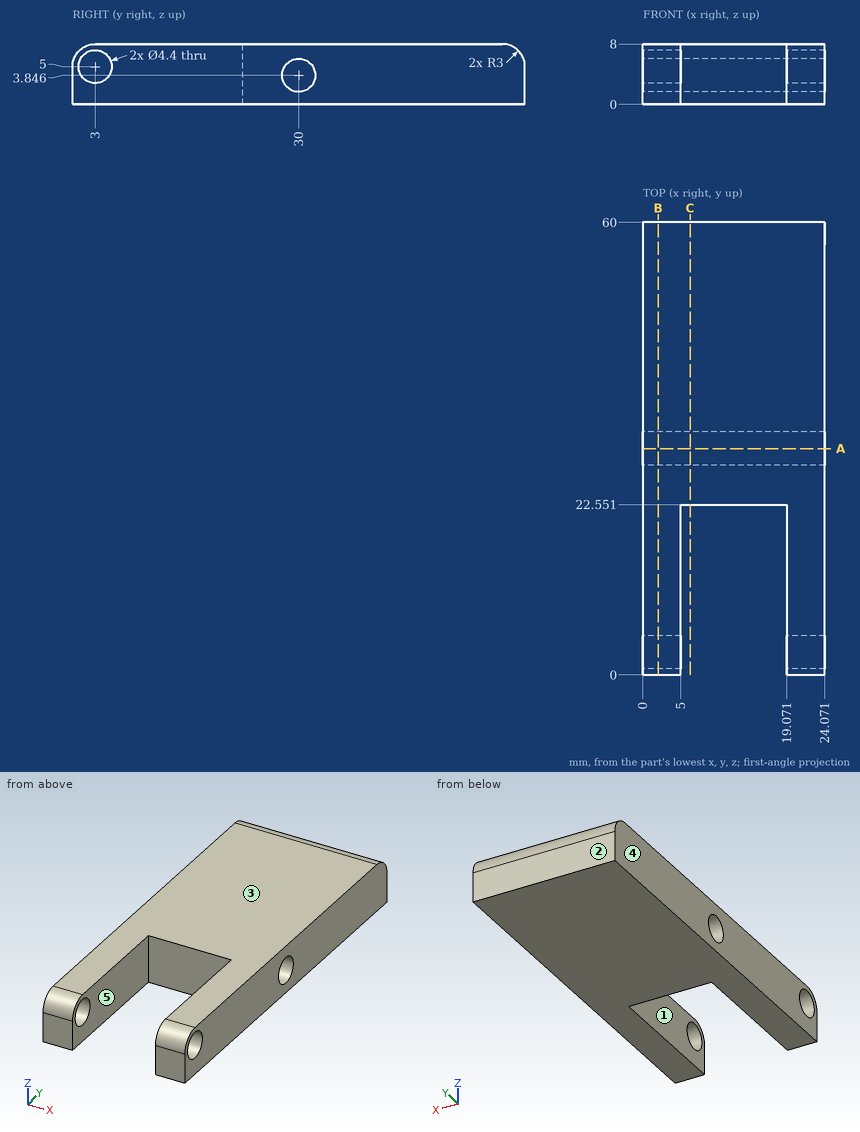
Answer from the drawing. Dimensions are ordinates in mm from the lowest x, y and z of the part. A direction names the side the tool comes from. Round coordinates to 2 decimals unless told otherwise and drop trailing zeros. Order: outer loops, then holes, each group sorted by start corner. A loop starts at its lowest first (then second) coordinate and runs counter-clockwise, first axis right, second up. Notation, with made-up numbers: (49.5, 4.5) - (56.5, 4.5) arc R27 ccw to (56.5, 39.5) - close; hole circle Ø9 at (30, 82). An arc over 180 degrees is marked (long way). Put each result on its own line as item: value. Start each with the question number.
(1) Find section A-A (y = 30). Give the vertices of the cut face in (x, z).
(2) For the marked faces 1 and 2, determine the directions among +Z, -Z, +X, -X, +Y, -Y from which every point of the face is accessible in a straight line to the end or side of a thin tool.
(3) Straight lines are drawn through the part: probe 1 along Z at (x, y) = (9.5, 30); probe 2 along Z at (x, y) = (23.05, 3); probe 3 along X at (y, z) = (7, 4.5). For each, find the intervals that lie inside material, in ascending order. Write a range as from..to.
(4) Determine the mould class of the marked faces 3, 4 and 5 for opening direction X: released by +X, released by -X, zero draft, split by the parting line, or undercut.
(5) Find section B-B (x = 2). Give the vertices of the cut face in (y, z), plus the area to 3 significant figures.
(6) Find section C-C (x = 6.25). Give the vertices of the cut face in (y, z).
(7) Given P1, Ø4, axis at y = 3, z = 5, coming from the -X side; P2, Ø1.5, axis at x = 14, z = 1.5, coming from the -Y side, each flat-ended and moving along its own axis, determine where each tip first touches the part or whether it passes through.
Reply:
1. outline: (0, 0) - (24.07, 0) - (24.07, 1.65) - (0, 1.65) - close; (0, 6.05) - (24.07, 6.05) - (24.07, 8) - (0, 8) - close
2. face 1: +Z, -Z, -Y
2. face 2: +Z, -Z, +X, -X, +Y
3. probe 1: 0..1.65, 6.05..8
3. probe 2: 0..2.8, 7.2..8
3. probe 3: 0..5, 19.07..24.07
4. face 3: zero draft
4. face 4: released by -X
4. face 5: undercut
5. outline: (0, 0) - (60, 0) - (60, 5) arc R3 ccw to (57, 8) - (3, 8) arc R3 ccw to (0, 5) - close; hole circle Ø4.4 at (3, 5); hole circle Ø4.4 at (30, 3.85)
5. area: 446 mm^2
6. outline: (22.55, 0) - (60, 0) - (60, 5) arc R3 ccw to (57, 8) - (22.55, 8) - close; hole circle Ø4.4 at (30, 3.85)
7. P1: through
7. P2: y = 22.55
